Study the drawing (mm; zero at the part's minimum x, y, z) and answer. A direction names the side the tool comes from. Coordinates: 2 decimals unless noted, no trailing zeros. Order: outer loops, then holes, each group sorted by start corner. A loop starts at its lowest first (then second) coordinate and runs counter-clockwise, first axis right, second up.
1. The part is cut by section C-C, the plane x = 6. Give the vertices of the cut face in (y, z), then the cut area to 3 significant figures.
2. The part is cut by section B-B, the plane x = 36. Give the vertices of the cut face in (y, z).
3. The part is cut by section A-A, the plane y = 46.65. Give the vertices of the cut face in (x, z), then the cut area to 3 significant figures.
4. A flat-ended cylindrical pin translates along its axis: pin 1 Ø8 at (y, z) = (23.5, 4) entering from +X. Find the tip coordinate at first contact, or state that the pin passes through.
5. A tool of negligible diameter and unlimited length cuts with its end or side. For the marked faces 4 and 5, from which of +Z, -Z, +X, -X, +Y, -Y can it reach the whole face along a straight path? Write none if from no direction.
6. Determine the mould class of the marked faces 1, 2 and 3 for opening direction X: +X half, -X half, draft (parallel to the pull), parting line (faces both ways), or undercut.
7. The part is cut by section D-D, the plane y = 28.65. Give the vertices of the cut face in (x, z).
8. Find the intervals of material crossed by probe 1 along Y at (x, z) = (19, 19); probe 2 along X at (y, z) = (1.95, 12.5); probe 3 along X at (y, z) = (1.3, 12.5), in increasing order.
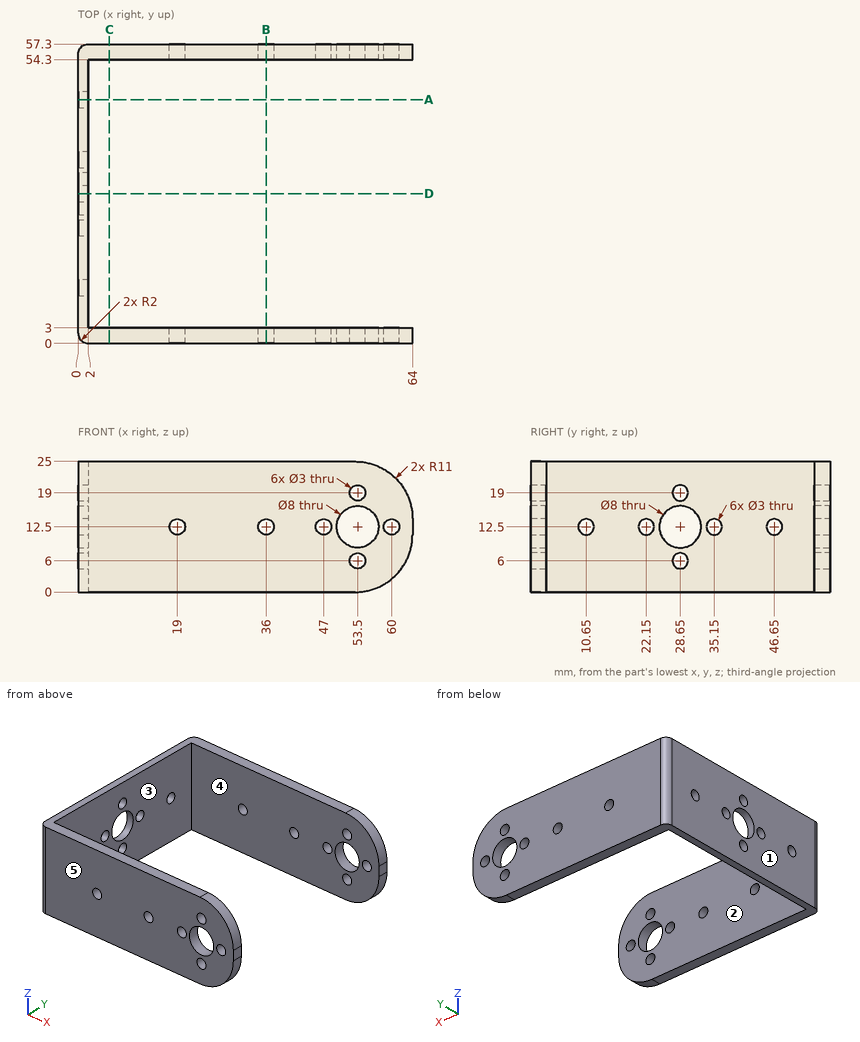
Geometry says:
1. outline: (0, 0) - (3, 0) - (3, 25) - (0, 25) - close; (54.3, 0) - (57.3, 0) - (57.3, 25) - (54.3, 25) - close
1. area: 150 mm2
2. outline: (0, 0) - (3, 0) - (3, 11) - (0, 11) - close; (0, 14) - (3, 14) - (3, 25) - (0, 25) - close; (54.3, 0) - (57.3, 0) - (57.3, 11) - (54.3, 11) - close; (54.3, 14) - (57.3, 14) - (57.3, 25) - (54.3, 25) - close
3. outline: (0, 0) - (2, 0) - (2, 11) - (0, 11) - close; (0, 14) - (2, 14) - (2, 25) - (0, 25) - close
3. area: 44.0 mm2
4. pin 1: stops at x = 2
5. face 4: +Z, -Z, +X
5. face 5: +Z, -Z, +X, -X, -Y
6. face 1: -X half
6. face 2: draft
6. face 3: +X half
7. outline: (0, 0) - (2, 0) - (2, 4.5) - (0, 4.5) - close; (0, 7.5) - (2, 7.5) - (2, 8.5) - (0, 8.5) - close; (0, 16.5) - (2, 16.5) - (2, 17.5) - (0, 17.5) - close; (0, 20.5) - (2, 20.5) - (2, 25) - (0, 25) - close
8. probe 1: y = 0 to 3, 54.3 to 57.3
8. probe 2: x = 0 to 17.5, 20.5 to 34.5, 37.5 to 45.5, 48.5 to 49.5, 57.5 to 58.5, 61.5 to 64
8. probe 3: x = 0.13 to 17.5, 20.5 to 34.5, 37.5 to 45.5, 48.5 to 49.5, 57.5 to 58.5, 61.5 to 64
